Read the model definition and answer for the solid it produces. Units are mm, in the model's axes. A direction names the side the tool comes from. Coordinates: 2 decimals unless noted, no trailing zeros. Write each loop counter-clockwise with the first axis right and the second up, starting at its lowest first coordinate (ties: lowest second). Pieces come first, ordered by that corner, then holes.
(1) Section A-A on z = 10 is taken. Write down the section's boundary in (x, y) (3 decimals).
(2) Which of the six approach directions +Z, -Z, +X, -X, +Y, -Y give full straight-line access (tool end or side, diameter ignored) to faces 1 (the flat face through (4, 9, -4.5)), 2 (the cylindrical face through (-3.1, 1, -10)), 3 (the flat face through (-0.7, 7, 8)), 4 (the flat face through (-1, 7.8, -5)), 5 (the flat face through (4, 1, 7.5))?
(3) Find the intervals of material crossed by probe 1 along X at (y, z) = (4.9, 10.05) (3 decimals); probe 2 along X at (y, z) = (8.95, -11); probe 3 along X at (y, z) = (1.4, 10), in increasing order.
(4) Given pin 1 (1.4 mm diameter, centred on x = -3.15, z = -11, fed in from +Y); pin 2 (2 mm diameter, centred on y = 1, z = 0.5, fed in from +X); pin 3 (1.8 mm diameter, centred on x = 4, y = 8.5, fed in from +Z), each flat-ended and moving along its own axis, determine where each tip first touches the part or whether it passes through.
(5) Section D-D on z = -11 is taken. Write down the section's boundary in (x, y), then the cut area to 3 significant figures.
(6) The mould has two halves that part along X. Classify faces 6 (the flat face through (-1, 2, 0)), 7 (the cylindrical face through (-4.22, 6.63, 9.96)), 8 (the flat face through (-0.7, 1, 2)): +X half, -X half, draft (parallel to the pull), parting line (faces both ways), or undercut.
(7) Section C-C on z = -8.25 is taken. Write down the section's boundary in (x, y), then the cut area to 3 significant figures.
(8) Section B-B on y = 4.9 is taken. Write down the section's boundary in (x, z) (3 decimals).
from build123d import *

# Parameters (mm, degrees)
SKETCH1_W                   = 12.6
SKETCH1_H                   = 25
BOSS_EXTRUDE1_DEPTH         = 10
SKETCH14_W                  = 7
SKETCH14_H                  = 5.8
CUT_EXTRUDE9_DEPTH          = 28.653028767
SKETCH15_W                  = 20
SKETCH15_H                  = 5.8
CUT_EXTRUDE10_DEPTH         = 18.47140521
CUT_EXTRUDE11_DEPTH         = 17.122654868
CUT_EXTRUDE11_DEPTH_BACK    = 17.122654868
SKETCH17_W                  = 7
SKETCH17_H                  = 12
SKETCH18_R                  = 1.875
CUT_EXTRUDE12_DEPTH         = 24.231228982
SKETCH19_W                  = 7
SKETCH19_H                  = 5
CUT_EXTRUDE13_DEPTH         = 2.2
FILLET2_R                   = 2
SKETCH20_R                  = 1
CUT_EXTRUDE18_DEPTH         = 5
TAP_DRILL_FOR_M2X0_4_TAP2_D = 1.6
M2_CLEARANCE_HOLE2_D        = 2.4


with BuildPart() as part:
    # Sketch1 → Boss-Extrude1 (new body)
    with BuildSketch(Plane(origin=(0, 0, 0), x_dir=(1, 0, 0), z_dir=(0, 1, 0))):
        Rectangle(SKETCH1_W, SKETCH1_H)
    extrude(amount=BOSS_EXTRUDE1_DEPTH)

    # Sketch14 → Cut-Extrude9 (cut, through all)
    with BuildSketch(Plane.XY.offset(12.5)):
        with Locations((2.8, 4.9)):
            Rectangle(SKETCH14_W, SKETCH14_H)
    extrude(amount=-CUT_EXTRUDE9_DEPTH, mode=Mode.SUBTRACT)

    # Sketch15 → Cut-Extrude10 (cut, through all)
    with BuildSketch(Plane(origin=(-0.7, 0, 0), x_dir=(0, 0, -1), z_dir=(1, 0, 0))):
        with Locations((2.5, 4.9)):
            Rectangle(SKETCH15_W, SKETCH15_H)
    extrude(amount=-CUT_EXTRUDE10_DEPTH, mode=Mode.SUBTRACT)

    # Sketch17 → Cut-Extrude11 (cut, two sides: drawn at the far end of the back side and taken through both)
    with BuildSketch(Plane(origin=(0, 2, 0), x_dir=(1, 0, 0), z_dir=(0, 1, 0)).offset(-CUT_EXTRUDE11_DEPTH_BACK)):
        with Locations((2.8, -1.5)):
            Rectangle(SKETCH17_W, SKETCH17_H)
    extrude(amount=CUT_EXTRUDE11_DEPTH + CUT_EXTRUDE11_DEPTH_BACK, mode=Mode.SUBTRACT)

    # Sketch18 → Cut-Extrude12 (cut, through all)
    with BuildSketch(Plane(origin=(0, 0, 7.5), x_dir=(-1, 0, 0), z_dir=(0, 0, -1))):
        with Locations(Location((3.5, 4.9, 0), (0, 0, 90))):
            Circle(SKETCH18_R)
    extrude(amount=-CUT_EXTRUDE12_DEPTH, mode=Mode.SUBTRACT)

    # Sketch19 → Cut-Extrude13 (cut)
    with BuildSketch(Plane(origin=(0, 10, 0), x_dir=(1, 0, 0), z_dir=(0, 1, 0))):
        with Locations((2.8, -10)):
            Rectangle(SKETCH19_W, SKETCH19_H)
    extrude(amount=-CUT_EXTRUDE13_DEPTH, mode=Mode.SUBTRACT)

    # Fillet2
    # the kernel refuses this fillet: 2 mm, written as the material it adds along each edge
    with BuildSketch(Plane(origin=(-0.7, 2, -4.5), x_dir=(1, 0, 0), z_dir=(0, -1, 0)), Plane(origin=(-0.7, 2, 7.5), x_dir=(0, 0, -1), z_dir=(0, -1, 0))) as fillet2_piece_1:
        with BuildLine():
            CenterArc((FILLET2_R, FILLET2_R), FILLET2_R, 180, 90)
            Line((0, FILLET2_R), (0, 0))
            Line((0, 0), (FILLET2_R, 0))
        make_face()
    extrude(amount=2)
    with BuildSketch(Plane(origin=(-0.7, 10, -4.5), x_dir=(1, 0, 0), z_dir=(0, -1, 0))) as fillet2_piece_2:
        with BuildLine():
            CenterArc((FILLET2_R, FILLET2_R), FILLET2_R, 180, 90)
            Line((0, FILLET2_R), (0, 0))
            Line((0, 0), (FILLET2_R, 0))
        make_face()
    extrude(amount=2.2)

    # Sketch20 → Cut-Extrude18 (cut)
    with BuildSketch(Plane.XZ):
        with Locations(Location((3.35, -11, 0), (0, 0, 270))):
            Circle(SKETCH20_R)
        with Locations(Location((-3.15, -11, 0), (0, 0, 270))):
            Circle(SKETCH20_R)
    extrude(amount=-CUT_EXTRUDE18_DEPTH, mode=Mode.SUBTRACT)

    # Tap Drill for M2x0.4 Tap2 (through all)
    with Locations(Plane(origin=(3.35, 10, -11), x_dir=(0, 0, 1), z_dir=(0, 1, 0))):
        with Locations((0, 0), (0, -6.5)):
            Hole(TAP_DRILL_FOR_M2X0_4_TAP2_D / 2)

    # M2 Clearance Hole2 (through all)
    with Locations(Plane(origin=(2.8, 2, 10), x_dir=(1, 0, 0), z_dir=(0, 1, 0))):
        with Locations((0, 0)):
            Hole(M2_CLEARANCE_HOLE2_D / 2)


solid = part.part
Response:
1. outline: (-6.3, 0) - (1.6, 0) - (1.6, 2) - (-0.7, 2) - (-0.7, 10) - (-6.3, 10) - close; (4, 0) - (6.3, 0) - (6.3, 2) - (4, 2) - close; hole circle Ø3.75 at (-3.5, 4.9)
2. face 1: +Z, +X, +Y, -Y
2. face 2: -Y
2. face 3: +Z, +X, +Y
2. face 4: -Z, +X, -X
2. face 5: +X, +Y, -Y
3. probe 1: x = -6.3 to -5.375, -1.625 to -0.7
3. probe 2: x = -6.3 to -3.95, -2.35 to 2.55, 4.15 to 6.3
3. probe 3: x = -6.3 to 1.6, 4 to 6.3
4. pin 1: passes through
4. pin 2: stops at x = -0.7
4. pin 3: stops at z = -4.5
5. outline: (-6.3, 0) - (-4.15, 0) - (-4.15, 2) - (-6.3, 2) - close; (-6.3, 7.8) - (-3.95, 7.8) - (-3.95, 10) - (-6.3, 10) - close; (-2.35, 7.8) - (2.55, 7.8) - (2.55, 10) - (-2.35, 10) - close; (-2.15, 0) - (2.35, 0) - (2.35, 2) - (-2.15, 2) - close; (4.15, 7.8) - (6.3, 7.8) - (6.3, 10) - (4.15, 10) - close; (4.35, 0) - (6.3, 0) - (6.3, 2) - (4.35, 2) - close
5. area: 37.9 mm2
6. face 6: draft
6. face 7: undercut
6. face 8: +X half
7. outline: (-6.3, 0) - (6.3, 0) - (6.3, 2) - (-6.3, 2) - close; (-6.3, 7.8) - (6.3, 7.8) - (6.3, 10) - (-6.3, 10) - close
7. area: 52.9 mm2
8. outline: (-6.3, 7.5) - (-5.375, 7.5) - (-5.375, 12.5) - (-6.3, 12.5) - close; (-1.625, 7.5) - (-0.7, 7.5) - (-0.7, 12.5) - (-1.625, 12.5) - close
